CAD build for the part. Positions are in the model's coordinates, mm. A direction names the side the tool comes from. Round coordinates to 2 decimals unless told otherwise and drop trailing zeros. Loops run counter-clockwise (first coordinate to the right, second up) from the corner with the lowest first, then second, coordinate; pieces in that order, holes last. Notation, with made-up numbers: M 75.5,-14.75 L 106.5,-14.75 A24 ccw 106.5,16.25 Z; hole C -17,9 d3. An arc over 180 degrees is marked long. Use a Markdown table: item, result. Add a question column.
(1) Band-saw the part on D-D, the plane z = 18. Write the cut outline in (x, y).
(2) Two-plate mould, pull along Z, no slides. Class faces 1 (the face through (0, -1, 26)), 2 (the face through (-0.105, 3.525, 23.095)), 3 (the face through (0, 2, 30)): released by +Z, released by -Z, zero draft, split by the parting line, or undercut.
(3) Band-saw the part on C-C, the plane y = 5.5. Write the cut outline in (x, z), and give its area (4 significant figures).
(4) Wall check: L1, parallel to Y at x = 0, z = 1.35; L2, parallel to X at y = 18, z = 1.95; L3, parallel to X at y = 5, z = 10. Give the ranges that are in metal, low to high.
(5) Band-saw the part on A-A, the plane y = 10. Write the cut outline in (x, z).
(6) Which spindle directions (+Z, -Z, +X, -X, +Y, -Y) get a long thin tool onto all of the face, cutting with end or side? Do faces 4 (the face through (-3, -0.5, 8)), 5 (the face through (0, -0.5, 27)), 6 (the face through (3, -0.5, 8)), 7 (the face through (4.832, 4.219, 15.463)). Say none if no direction does.
(7) Flat gauge pins, fed straight in: P1, Ø0.5, axis at x = 0, y = -0.5, coming from the +Z side; P2, Ø4, axis at x = 0, z = 18, coming from the +Y side; P3, Ø0.5, axis at y = -0.5, z = 8, coming from the +X side; P4, Ø8.5, axis at x = 0, y = 10, coming from the +Z side. Where does each tip first touch, or does it go through?
(8) Band-saw the part on B-B, the plane x = 0. Give the number of separate pieces and of enclosed holes in the cut face, and give its area (3 significant figures).
Autodesk Inventor part; units mm, degrees
ref_plane "bracket_to_bolt_XY" through (1, 10, 0) normal (0, 0, 1) x (1, 0, 0)
ref_plane "bracket_to_bolt_YZ" through (1, 10, 0) normal (1, 0, 0) x (0, 1, 0)
ref_plane "bracket_to_bolt_ZX" through (1, 10, 0) normal (0, 1, 0) x (0, 0, 1)
sketch "Sketch_15" plane through (0, 0, 0) normal (1, 0, 0) x (0, 1, 0)
  line L0 (0, 30) -> (0, 0)
  line L1 (0, 0) -> (30, 0)
  line L2 (30, 0) -> (30, 4.0858)
  arc A0 (30, 4.0858) -> (29.7071, 4.7929) centre (29, 4.0858) ccw
  line L3 (29.7071, 4.7929) -> (4.7929, 29.7071)
  arc A1 (4.7929, 29.7071) -> (4.0858, 30) centre (4.0858, 29) ccw
  line L4 (4.0858, 30) -> (0, 30)
extrude "Extrusion1" add sketch "Sketch_15" along normal mid plane 20
sketch "Sketch_16" plane through (0, 0, 0) normal (1, 0, 0) x (0, 1, 0)
  line L0 (2.9278, 34.5) -> (4.5, 4.5)
  line L1 (4.5, 4.5) -> (34.5, 4.5)
  line L2 (34.5, 4.5) -> (34.5, 34.5)
  line L3 (34.5, 34.5) -> (2.9278, 34.5)
extrude "Extrusion2" cut sketch "Sketch_16" along normal mid plane 15
sketch "Sketch_17" plane through (0, 4.5, 0) normal (0, 1, 0) x (1, 0, 0)
  line L0 (-5.4209, -10.5) -> (-4.4687, -18.5299)
  arc A0 (-4.4687, -18.5299) -> (4.4687, -18.5299) centre (0, -18) ccw
  line L1 (4.4687, -18.5299) -> (5.4209, -10.5)
  line L2 (5.4209, -10.5) -> (-5.4209, -10.5)
extrude "Extrusion3" add sketch "Sketch_17" against normal blind 2.25
sketch "Sketch4" plane through (10, 0, 0) normal (0, 0, -1) x (-1, 0, 0)
  point P0 (10, 18)
hole "Hole1" at (0, 18, 0) direction (0, 0, 1) diameter 5.2 depth 4.5
sketch "Sketch5" plane through (10, 0, 0) normal (0, 0, -1) x (-1, 0, 0)
  point P0 (10, 10)
hole "Hole2" at (0, 10, 0) direction (0, 0, 1) diameter 5.2 depth 4.5
sketch "Sketch6" plane through (-10, 0, 30) normal (0, -1, 0) x (1, 0, 0)
  point P0 (10, -12)
hole "Hole3" at (0, 0, 18) direction (0, 1, 0) diameter 5.2 depth 4.5
sketch "Sketch_1" plane through (0, 0, 0) normal (0, 1, 0) x (-1, 0, 0)
  line L0 (10, 0) -> (10, 30)
  line L1 (10, 30) -> (-10, 30)
  line L2 (-10, 30) -> (-10, 0)
  line L3 (-10, 0) -> (10, 0)
extrude "Extrusion4" add sketch "Sketch_1" against normal blind 1
sketch "Sketch_4" plane through (0, 0, 0) normal (0, 1, 0) x (-1, 0, 0)
  line L0 (10, 0) -> (10, 30)
  line L1 (10, 30) -> (-10, 30)
  line L2 (-10, 30) -> (-10, 0)
  line L3 (-10, 0) -> (10, 0)
  arc A0 (3, 10.7) -> (2.7, 11) centre (2.7, 10.7) ccw
  line L4 (2.7, 11) -> (-2.7, 11)
  arc A1 (-2.7, 11) -> (-3, 10.7) centre (-2.7, 10.7) ccw
  line L5 (-3, 10.7) -> (-3, 5.3)
  arc A2 (-3, 5.3) -> (-2.7, 5) centre (-2.7, 5.3) ccw
  line L6 (-2.7, 5) -> (2.7, 5)
  arc A3 (2.7, 5) -> (3, 5.3) centre (2.7, 5.3) ccw
  line L7 (3, 5.3) -> (3, 10.7)
  arc A4 (3, 26.7) -> (2.7, 27) centre (2.7, 26.7) ccw
  line L8 (2.7, 27) -> (-2.7, 27)
  arc A5 (-2.7, 27) -> (-3, 26.7) centre (-2.7, 26.7) ccw
  line L9 (-3, 26.7) -> (-3, 24.3)
  arc A6 (-3, 24.3) -> (-2.7, 24) centre (-2.7, 24.3) ccw
  line L10 (-2.7, 24) -> (2.7, 24)
  arc A7 (2.7, 24) -> (3, 24.3) centre (2.7, 24.3) ccw
  line L11 (3, 24.3) -> (3, 26.7)
extrude "Extrusion5" cut sketch "Sketch_4" against normal blind 1
ref_plane "bracket_to_bolt_XY" through (1, 10, 0) normal (0, 0, 1) x (1, 0, 0)
ref_plane "bracket_to_bolt_YZ" through (1, 10, 0) normal (1, 0, 0) x (0, 1, 0)
ref_plane "bracket_to_bolt_ZX" through (1, 10, 0) normal (0, 1, 0) x (0, 0, 1)
ref_plane "bracket_to_dummy_XY" through (0, 0, 0) normal (0, 1, 0) x (1, 0, 0)
ref_plane "bracket_to_dummy_YZ" through (0, 0, 0) normal (1, 0, 0) x (0, 0, -1)
ref_plane "bracket_to_dummy_ZX" through (0, 0, 0) normal (0, 0, -1) x (0, 1, 0)
ref_plane "to_bolt_4_7_base_XY" through (0, 4.5, 18) normal (0, 1, 0) x (1, 0, 0)
ref_plane "to_bolt_4_7_base_YZ" through (0, 4.5, 18) normal (1, 0, 0) x (0, 0, -1)
ref_plane "to_bolt_4_7_base_ZX" through (0, 4.5, 18) normal (0, 0, -1) x (0, 1, 0)
ref_plane "to_bolt_row_4_to_7_XY" through (0, 18, 4.5) normal (0, 0, 1) x (1, 0, 0)
ref_plane "to_bolt_row_4_to_7_YZ" through (0, 18, 4.5) normal (1, 0, 0) x (0, 1, 0)
ref_plane "to_bolt_row_4_to_7_ZX" through (0, 18, 4.5) normal (0, 1, 0) x (0, 0, 1)
ref_plane "to_nut_base_4_7_XY" through (0, -2, 18) normal (0, 1, 0) x (1, 0, 0)
ref_plane "to_nut_base_4_7_YZ" through (0, -2, 18) normal (1, 0, 0) x (0, 0, -1)
ref_plane "to_nut_base_4_7_ZX" through (0, -2, 18) normal (0, 0, -1) x (0, 1, 0)
ref_plane "to_nut_row_4_to_7_XY" through (0, 18, -2) normal (0, 0, 1) x (1, 0, 0)
ref_plane "to_nut_row_4_to_7_YZ" through (0, 18, -2) normal (1, 0, 0) x (0, 1, 0)
ref_plane "to_nut_row_4_to_7_ZX" through (0, 18, -2) normal (0, 1, 0) x (0, 0, 1)
properties part number "HBLFSNK5hblfsn5" material "アルミニウム 6061"
Return value:
| question | item | result |
|---|---|---|
| 1 | outline | M -10,0 L -2.6,0 L -2.6,4.5 L -4.53,4.5 L -4.53,3.79 L -7.5,3.79 L -7.5,16.5 L -10,16.5 Z; M 2.6,0 L 10,0 L 10,16.5 L 7.5,16.5 L 7.5,3.79 L 4.53,3.79 L 4.53,4.5 L 2.6,4.5 Z |
| 2 | face 1 | zero draft |
| 2 | face 2 | undercut |
| 2 | face 3 | released by +Z |
| 3 | outline | M -10,0 L 10,0 L 10,29 L 7.5,29 L 7.5,4.5 L -7.5,4.5 L -7.5,29 L -10,29 Z |
| 3 | area | 212.5 mm^2 |
| 4 | L1 | 0 to 7.4, 12.6 to 15.4, 20.6 to 30 |
| 4 | L2 | -10 to -2.6, 2.6 to 10 |
| 4 | L3 | -10 to -7.5, 7.5 to 10 |
| 5 | outline | M -10,0 L -2.6,0 L -2.6,4.5 L -7.5,4.5 L -7.5,24.5 L -10,24.5 Z; M 2.6,0 L 10,0 L 10,24.5 L 7.5,24.5 L 7.5,4.5 L 2.6,4.5 Z |
| 6 | face 4 | +Z, -Z, -X, -Y |
| 6 | face 5 | +Z, +X, -X, -Y |
| 6 | face 6 | +Z, -Z, +X, -Y |
| 6 | face 7 | +Z, +Y |
| 7 | P1 | z = 27 |
| 7 | P2 | through |
| 7 | P3 | x = 3 |
| 7 | P4 | z = 4.5 |
| 8 | separate pieces | 4 |
| 8 | enclosed holes | 0 |
| 8 | area | 179 mm^2 |
